Here's how the part is built. I have some questions about the finished solid (model axes, mm). Face numbers are marked on the shaded views. A direction names the side the tool comes from. Coordinates: 2 decimals unless noted, no trailing zeros. Write each loop counter-clockwise with the first axis right and the second up, starting at its lowest first coordinate (ties: lowest second). Pieces come first, ordered by that corner, then holes.
Item 1: For the marked faces 1 and 2, which set-ups out of +Z, -Z, +X, -X, +Y, -Y let a thin tool reach every point of the face, with its end or its side?
Item 2: Please list where these lines run through material, in increasing order: line 1 (Z direction, x = -4, y = 53); line 2 (Y direction, x = 5.5, z = 22.25); line 3 (X direction, y = 13, z = 2.25).
Item 3: I want a section at C-C (z = 8.25). Please give me the cut outline in (x, y).
Item 4: I want a section at A-A (y = 0). Please give me the cut outline in (x, z).
Item 5: I'm going to push flat-ended pins straight in: P1, Ø5, axis at x = -23.5, y = 49, coming from the -Z side; P2, Ø10, axis at x = 36.5, z = 6, coming from the +Y side; P3, Ø3, axis at x = 26, z = 5, coming from the -Y side; P4, Ø1.5, axis at y = 8.5, z = 11.5, coming from the +X side. Where does each tip first touch, or does it pass through?
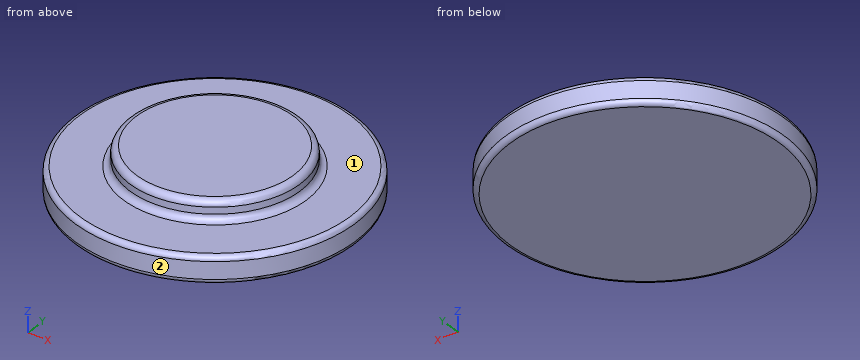
from build123d import *

# Parameters (mm, degrees)
F0_R     = 75.672097
F1_DEPTH = 14.57094
F2_R     = 45.928077
F3_DEPTH = 10.490498
F4_R     = 3.436595
F5_R     = 2.666092


with BuildPart() as f1:
    # F0 (on Top) → F1 (new body)
    with BuildSketch(Plane.XY):
        Circle(F0_R)
    extrude(amount=F1_DEPTH)

    # F2 (on face) → F3 (join)
    with BuildSketch(Plane.XY.offset(14.57094)):
        Circle(F2_R)
    extrude(amount=F3_DEPTH)

    # F4
    f4_edges = [f1.edges().sort_by_distance(p)[0] for p in [
        (45.928077, 0, 19.816189),
        (-45.928077, 0, 14.57094),
        (-45.928077, 0, 25.061438),
    ]]
    fillet(f4_edges, radius=F4_R)

    # F5
    f5_edges = [f1.edges().sort_by_distance(p)[0] for p in [
        (75.672097, 0, 7.28547),
        (-75.672097, 0, 0),
        (-75.672097, 0, 14.57094),
    ]]
    fillet(f5_edges, radius=F5_R)


solid = f1.part
Answer:
1. face 1: +Z
1. face 2: +Z, -Z
2. line 1: z = 0 to 14.57
2. line 2: y = -45.54 to 45.54
2. line 3: x = -74.51 to 74.51
3. outline: circle Ø151.34 at (0, 0)
4. outline: (-75.67, 2.67) arc R2.67 ccw to (-73.01, 0) - (73.01, 0) arc R2.67 ccw to (75.67, 2.67) - (75.67, 11.9) arc R2.67 ccw to (73.01, 14.57) - (49.36, 14.57) arc R3.44 cw to (45.93, 18.01) - (45.93, 21.62) arc R3.44 ccw to (42.49, 25.06) - (-42.49, 25.06) arc R3.44 ccw to (-45.93, 21.62) - (-45.93, 18.01) arc R3.44 cw to (-49.36, 14.57) - (-73.01, 14.57) arc R2.67 ccw to (-75.67, 11.9) - close
5. P1: stops at z = 0
5. P2: stops at y = 68.8
5. P3: stops at y = -71.6
5. P4: stops at x = 75.27
